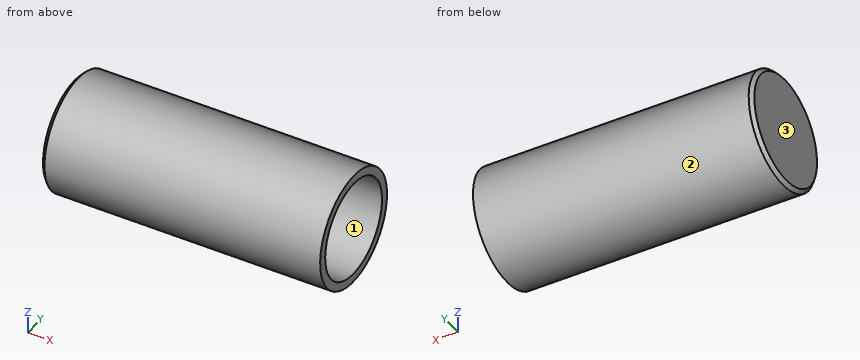
```python
from build123d import *

# Parameters (mm, degrees)
SKETCH_2_W     = 39
SKETCH_2_H     = 8
SHELL_4_T      = -1.2
CHAMFER_2_SIZE = 0.5


with BuildPart() as part:
    # 草图2 → 旋转2 (revolve)
    with BuildSketch(Plane(origin=(0, 17.555203641, 0), x_dir=(1, 0, 0), z_dir=(0, 0, 1)), mode=Mode.PRIVATE) as revolve_2_sk:
        with Locations((21.172378693, 10.620939958)):
            Rectangle(SKETCH_2_W, SKETCH_2_H)
    revolve(revolve_2_sk.sketch.rotate(Axis((1.672378693, 24.176143599, 0), (1, 0, 0)), 90), axis=Axis((1.672378693, 24.176143599, 0), (1, 0, 0)))

    # 抽壳4
    shell_4_openings = [part.faces().sort_by_distance(p)[0] for p in [
        (40.672378693, 24.176143599, 0),
    ]]
    offset(amount=SHELL_4_T, openings=shell_4_openings, kind=Kind.INTERSECTION)

    # 倒角2
    chamfer_2_edges = [part.edges().sort_by_distance(p)[0] for p in [
        (2.872378693, 24.176143599, -6.8),
        (1.672378693, 24.176143599, -8),
    ]]
    chamfer(chamfer_2_edges, length=CHAMFER_2_SIZE)


solid = part.part
```
Verification items for the finished model (mm, model axes). Face numbers are marked on the shaded views. Give positions to 0.01 mm unless a question says otherwise; leave off trailing zeros. Loops run counter-clockwise (first coordinate to the right, second up) from the corner with the lowest first, then second, coordinate; pieces in that order, holes last. Notation, with made-up numbers: M -29.5,53.5 L 13.5,53.5 A17 cw 13.5,73.5 Z; hole C -8,15.25 d9. An arc over 180 degrees is marked long. Return JSON: item names as keys, results as strings.
1) Section check B-B, the plane x = 11. Enter the section's corners in (y, z), and give its area (3 significant figures).
Findings:
{"outline": "C 24.18,0 d16; hole C 24.18,0 d13.6", "area": "55.8 mm2"}
2) Mould release check, pull along Y, two halves, no side actions. Record for the marked faces 1, 2 and 3: released by +Y, released by -Y, zero draft, split by the parting line, or undercut.
Findings:
{"face 1": "undercut", "face 2": "split by the parting line", "face 3": "zero draft"}
3) Gauge pin test, flat ends, axial feed: P1, Ø4, axis at x = 18.5, z = 6, coming from the -Y side; P2, Ø5, axis at x = 36.5, y = 28.5, coming from the -Z side. Record the tip position at first contact, or that the pin passes through.
Findings:
{"P1": "stops at y = 17.25", "P2": "stops at z = -7.79"}
4) Section check A-A, the plane z = 0. Enter the section's corners in (x, y).
Findings:
{"outline": "M 1.67,16.68 L 2.17,16.18 L 40.67,16.18 L 40.67,17.38 L 3.37,17.38 L 2.87,17.88 L 2.87,30.48 L 3.37,30.98 L 40.67,30.98 L 40.67,32.18 L 2.17,32.18 L 1.67,31.68 Z"}
5) Material ranges on L1, parallel to Z at x = 11, y = 24.25; L2, parallel to Y at x = 26, z = 0; L3, parallel to X at y = 26.5, z = 2.25, recorded low to high. Write a range as [from, to].
Findings:
{"L1": "z = [-8, -6.8], [6.8, 8]", "L2": "y = [16.18, 17.38], [30.98, 32.18]", "L3": "x = [1.67, 2.87]"}
